```python
from build123d import *

# Parameters (mm, degrees)
F0_R      = 33.5
F1_DEPTH  = 20
F2_R      = 32.5
F3_DEPTH  = 18
F4_R      = 10.5
F5_DEPTH  = 11
F6_R      = 9.5
F7_DEPTH  = 9.9
F8_R      = 9
F9_DEPTH  = 17
F10_R     = 12
F11_DEPTH = 2
F11_TAPER = 70
F12_DEPTH = 5


with BuildPart() as f1:
    # F0 (on Top) → F1 (new body)
    with BuildSketch(Plane.XY):
        Circle(F0_R)
    extrude(amount=F1_DEPTH)

    # F2 (on face) → F3 (cut)
    with BuildSketch(Plane(origin=(0, 0, 0), x_dir=(1, 0, 0), z_dir=(0, 0, -1))):
        Circle(F2_R)
    extrude(amount=-F3_DEPTH, mode=Mode.SUBTRACT)

    # F4 (on face) → F5 (join)
    with BuildSketch(Plane.XY.offset(20)):
        Circle(F4_R)
    extrude(amount=F5_DEPTH)

    # F6 (on face) → F7 (cut)
    with BuildSketch(Plane.XY.offset(31)):
        Circle(F6_R)
    extrude(amount=-F7_DEPTH, mode=Mode.SUBTRACT)

    # F8 (on face) → F9 (join)
    with BuildSketch(Plane.XY.offset(21.1)):
        Circle(F8_R)
    extrude(amount=F9_DEPTH)

    # F10 (on face) → F11 (join)
    with BuildSketch(Plane.XY.offset(38.1)):
        Circle(F10_R)
    extrude(amount=F11_DEPTH, taper=F11_TAPER)

    # F12 (cut): a face of the model
    f12_faces = [f1.faces().sort_by_distance(p)[0] for p in [
        (0, 0, 40.1),
    ]]
    extrude(f12_faces, amount=-F12_DEPTH, mode=Mode.SUBTRACT)


solid = f1.part
```
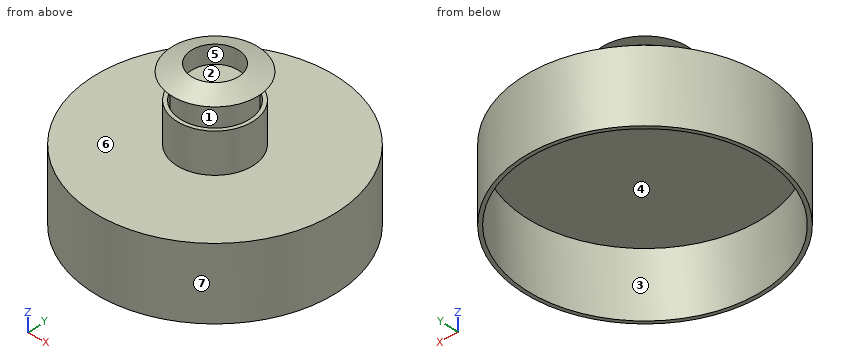
Build history of the part. All positions in model axes, mm. Face numbers are marked on the shaded views. A direction names the side the tool comes from. Round coordinates to 2 decimals unless told otherwise and drop trailing zeros. Write each loop counter-clockwise with the first axis right and the second up, starting at its lowest first coordinate (ties: lowest second). Pieces come first, ordered by that corner, then holes. Notation, with made-up numbers: (-26, 64.25) -> (5, 64.25) arc R17 ccw to (5, 94.25) -> close; hole circle Ø4 at (85, 83). An arc over 180 degrees is marked (long way). Put each result on its own line as item: value.
Item 1: Two-plate mould, pull along Y, no slides. Class the marked faces 4, 5, 6 and 7: pulls with the +Y half, pulls with the -Y half, needs draft (parallel to the pull), parting line crosses it, or undercut.
Here are the results:
face 4: undercut
face 5: undercut
face 6: needs draft
face 7: parting line crosses it
Item 2: Wall check: probe 1 along Y at (x, z) = (0, 24.5); probe 2 along Y at (x, z) = (0, 37); probe 3 along Y at (x, z) = (0, 13). Give the ranges that are in metal, low to high. Write a range as from..to.
Here are the results:
probe 1: y = -10.5..-9.5, -9..9, 9.5..10.5
probe 2: y = -9..-6.51, 6.51..9
probe 3: y = -33.5..-32.5, 32.5..33.5
Item 3: Slice it at A-A, the plane z = 28. Give the cut face in (x, y), plus the area to 3 significant figures.
Here are the results:
outline: circle Ø21 at (0, 0); circle Ø18 at (0, 0); hole circle Ø19 at (0, 0)
area: 317 mm^2
Item 4: Flat gauge pins, fed straight in: P1, Ø15, axis at x = 0, y = 0, coming from the -Z side; P2, Ø8, axis at x = 17, y = -8.5, coming from the +Z side; P3, Ø5, axis at x = -5, z = 6, coming from the -Y side. Where does each tip first touch, or does it go through?
Here are the results:
P1: stops at z = 18
P2: stops at z = 20
P3: stops at y = -33.41
Item 5: Slice it at B-B, the plane y = 0. Give the cut face in (x, z).
Here are the results:
outline: (-33.5, 0) -> (-32.5, 0) -> (-32.5, 18) -> (32.5, 18) -> (32.5, 0) -> (33.5, 0) -> (33.5, 20) -> (10.5, 20) -> (10.5, 31) -> (9.5, 31) -> (9.5, 21.1) -> (9, 21.1) -> (9, 38.1) -> (12, 38.1) -> (6.51, 40.1) -> (6.51, 35.1) -> (-6.51, 35.1) -> (-6.51, 40.1) -> (-12, 38.1) -> (-9, 38.1) -> (-9, 21.1) -> (-9.5, 21.1) -> (-9.5, 31) -> (-10.5, 31) -> (-10.5, 20) -> (-33.5, 20) -> close
Item 6: Tool access for the marked faces 1, 2 and 3: list every direction of +Z, -Z, +X, -X, +Y, -Y with a clear straight run to the whole face (end or side of a thin tool).
Here are the results:
face 1: none
face 2: +Z
face 3: -Z
Item 7: Slice it at D-D, the plane z = 3. Give the cut face in (x, y).
Here are the results:
outline: circle Ø67 at (0, 0); hole circle Ø65 at (0, 0)
